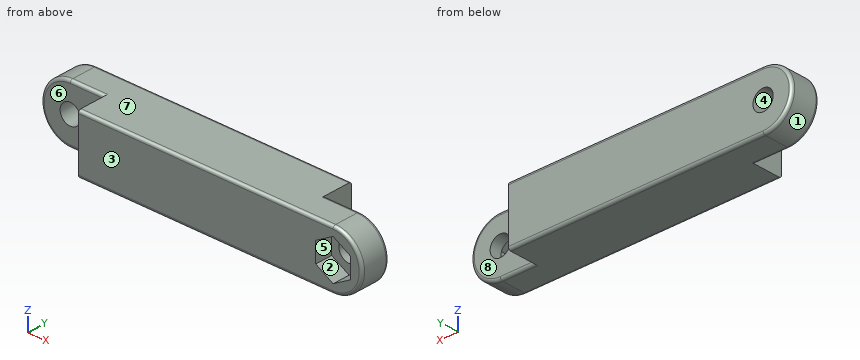
from build123d import *

# Parameters (mm, degrees)
F0_W     = 50
F0_H     = 10
F1_DEPTH = 10
F2_W     = 13.4624946701
F2_H     = 5
F2_W_2   = 13.2752915323
F3_DEPTH = 25
F4_R     = 1.75
F5_DEPTH = 25
F7_DEPTH = 3
F8_R     = 0.5


# Not quite as in the source:
# - a feature names something its author has since deleted; it is built from what else it names


with BuildPart() as f1:
    # F0 (on Front) → F1 (new body)
    with BuildSketch(Plane.XZ):
        with Locations((25, 5)):
            Rectangle(F0_W, F0_H)
        with BuildLine():
            ThreePointArc((0, 10), (-5, 5), (0, 0))
            Line((0, 0), (0, 10))
        make_face()
        with BuildLine():
            Line((50, 10), (50, 0))
            ThreePointArc((50, 0), (55, 5), (50, 10))
        make_face()
    extrude(amount=F1_DEPTH)

    # F2 (on face) → F3 (cut)
    with BuildSketch(Plane.XY.offset(10)):
        with Locations((-0.7312473351, -7.5)):
            Rectangle(F2_W, F2_H)
        with Locations((50.6376457661, -2.5)):
            Rectangle(F2_W_2, F2_H)
    extrude(amount=-F3_DEPTH, mode=Mode.SUBTRACT)

    # F4 (on face) → F5 (cut)
    with BuildSketch(Plane.XZ.offset(10)):
        with Locations((50, 5)):
            Circle(F4_R)
        with Locations((0, 5)):
            Circle(F4_R)
    extrude(amount=-F5_DEPTH, mode=Mode.SUBTRACT)

    # F6 (on face) → F7 (cut)
    with BuildSketch(Plane.XZ.offset(10)):
        Polygon((53, 3.2679491924), (53, 6.7320508076), (50, 8.4641016151), (47, 6.7320508076), (47, 3.2679491924), (50, 1.5358983849), align=None)
    extrude(amount=-F7_DEPTH, mode=Mode.SUBTRACT)

    # F8
    f8_edges = [f1.edges().sort_by_distance(p)[0] for p in [
        (28, -10, 10),
        (22, 0, 10),
        (-5, -5, 5),
        (55, -5, 5),
        (22, 0, 0),
        (47, -5, 0),
        (28, -10, 0),
        (3, -5, 0),
        (-5, 0, 5),
        (47, -5, 10),
        (55, -10, 5),
        (3, -5, 10),
    ]]
    fillet(f8_edges, radius=F8_R)


solid = f1.part
Source: CAD feature listing. Evaluate the final solid. Frame: model axes, mm. Face numbers are marked on the shaded views. A direction names the side the tool comes from. Coordinates: 2 decimals unless noted, no trailing zeros. Loops run counter-clockwise (first coordinate to the right, second up) from the corner with the lowest first, then second, coordinate; pieces in that order, holes last. Notation, with made-up numbers: M 41.5,24 L 90.5,24 A19 cw 90.5,36 Z; hole C 56,63 d4. An arc over 180 degrees is marked long. Answer in a Markdown table with one row per item.
Q1. Set-up query: the marked faces 4, 5, 6, 7 and 8. Return all of +Z, -Z, +X, -X, +Y, -Y with unobstructed straight access to the full face (end or side cutting, diameter ignored); none if empty.
Answers below:
| item | result |
|---|---|
| face 4 | +Y, -Y |
| face 5 | -Y |
| face 6 | +Z, -Z, -X, -Y |
| face 7 | +Z, +X, -X, +Y, -Y |
| face 8 | +Z, -Z, +X, +Y |
Q2. Section D-D on y = -1. Return the cut outline in (x, z), plus the area to 3 significant figures.
Answers below:
| item | result |
|---|---|
| outline | M 0,0 L 44,0 L 44,10 L 0,10 A5 ccw Z; hole C 0,5 d3.5 |
| area | 470 mm^2 |
Q3. Section B-B on y = -8. Return the cut outline in (x, z), plus the area to 3 significant figures.
Answers below:
| item | result |
|---|---|
| outline | M 6,0 L 50,0 A5 ccw 50,10 L 6,10 Z; hole M 47,3.27 L 50,1.54 L 53,3.27 L 53,6.73 L 50,8.46 L 47,6.73 Z |
| area | 448 mm^2 |
Q4. Section A-A on z = 5. Return the cut outline in (x, y).
Answers below:
| item | result |
|---|---|
| outline | M -5,-4.5 A0.5 ccw -4.5,-5 L -1.75,-5 L -1.75,0 L -4.5,0 A0.5 ccw -5,-0.5 Z; M 1.75,-5 L 6,-5 L 6,-10 L 47,-10 L 47,-7 L 48.25,-7 L 48.25,-5 L 44,-5 L 44,0 L 1.75,0 Z; M 51.75,-7 L 53,-7 L 53,-10 L 54.5,-10 A0.5 ccw 55,-9.5 L 55,-5.5 A0.5 ccw 54.5,-5 L 51.75,-5 Z |
Q5. Ray query, probe 1 along Z at (x, y) = (0, -1.1); probe 2 along X at (y, z) = (-8, 6); probe 3 along Y at (x, z) = (5.5, 1.5). Return the intervals inside material, ascending. Write a range as from..to.
Answers below:
| item | result |
|---|---|
| probe 1 | z = 0..3.25, 6.75..10 |
| probe 2 | x = 6..47, 53..54.9 |
| probe 3 | y = -5..0 |
Q6. Section C-C on x = 5. Return the cut outline in (y, z), plus the area to 3 significant figures.
Answers below:
| item | result |
|---|---|
| outline | M -5,0.5 A0.5 ccw -4.5,0 L -0.5,0 A0.5 ccw 0,0.5 L 0,9.5 A0.5 ccw -0.5,10 L -4.5,10 A0.5 ccw -5,9.5 Z |
| area | 49.8 mm^2 |
Q7. First-contact query: pin 1 (2 mm diameter, centred on y = -6.5, z = 2, fed in from -X); pin 2 (4.5 mm diameter, centred on x = 50.5, z = 5.5, fed in from +Y); pin 3 (1 mm diameter, centred on y = -3.5, z = 8, fed in from +X). Flat tips, straight axial feed; report the tip coordinate or a pass-through.
Answers below:
| item | result |
|---|---|
| pin 1 | stops at x = 6 |
| pin 2 | stops at y = -5 |
| pin 3 | stops at x = 44 |
Q8. Draft query along Z for the marked faces 1, 2 and 3. Return one class per face: pulls with the +Z half, pulls with the -Z half, needs draft (parallel to the pull), parting line crosses it, or undercut.
Answers below:
| item | result |
|---|---|
| face 1 | parting line crosses it |
| face 2 | undercut |
| face 3 | needs draft |
